Work out the finished part from the listing and answer in its coordinate system (mm). Face numbers are marked on the shaded views. Round coordinates to 2 decimals unless told otherwise and drop trailing zeros. Order: outer loops, then holes, each group sorted by start corner. A loop starts at its lowest first (then second) coordinate and runs counter-clockwise, first axis right, second up. Notation, with made-up numbers: (-30.75, 78.5) - (10.25, 78.5) arc R20 cw to (10.25, 113.5) - close; hole circle Ø4 at (29, 61). An arc over 180 degrees is marked (long way). Use CSV: the item, a comma, the result in double quotes.
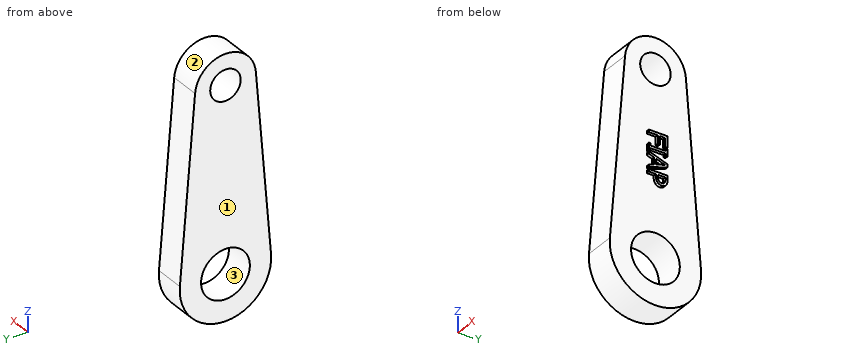
Autodesk Inventor part; units mm, degrees
ref_plane "YZ Plane" through (0, 0, 0) normal (1, 0, 0) x (0, 1, 0)
ref_plane "XZ Plane" through (0, 0, 0) normal (0, 1, 0) x (-1, 0, 0)
ref_plane "XY Plane" through (0, 0, 0) normal (0, 0, 1) x (1, 0, 0)
sketch "Esboço1" plane through (0, 0, 0) normal (1, 0, 0) x (0, 1, 0)
  line L0 (0, 0) -> (0, 30)
  circle A0 centre (0, 0) radius 4
  circle A1 centre (0, 30) radius 2.5
  arc A2 (4.9826, 30.4167) -> (-4.9826, 30.4167) centre (0, 30) ccw
  arc A3 (-7.4739, 0.625) -> (7.4739, 0.625) centre (0, 0) ccw
  line L1 (4.9826, 30.4167) -> (7.4739, 0.625)
  line L2 (-4.9826, 30.4167) -> (-7.4739, 0.625)
extrude "Extrusão1" add sketch "Esboço1" along normal mid plane 5
sketch "Esboço2" plane through (2.5, 0, 0) normal (1, 0, 0) x (0, 0, -1)
  line L0 (-19.9846, 1.6224) -> (-11.4087, 1.6224) construction
  line L1 (-11.4087, 1.6224) -> (-11.4087, -1.4256) construction
  line L2 (-11.4087, -1.4256) -> (-19.9846, -1.4256) construction
  line L3 (-19.9846, -1.4256) -> (-19.9846, 1.6224) construction
  circle A0 centre (-30, 0) radius 2.5
  line L4 (-17.853, 1.2618) -> (-19.2708, 1.2618)
  line L5 (-19.2708, 1.2618) -> (-19.2708, 0.4022)
  line L6 (-19.2708, 0.4022) -> (-17.9122, 0.4022)
  line L7 (-17.9122, 0.4022) -> (-17.9122, 0.0416)
  line L8 (-17.9122, 0.0416) -> (-19.2708, 0.0416)
  line L9 (-19.2708, 0.0416) -> (-19.2708, -1.4256)
  line L10 (-19.2708, -1.4256) -> (-19.6758, -1.4256)
  line L11 (-19.6758, -1.4256) -> (-19.6758, 1.6224)
  line L12 (-19.6758, 1.6224) -> (-17.853, 1.6224)
  line L13 (-17.853, 1.6224) -> (-17.853, 1.2618)
  line L14 (-16.4278, -1.4256) -> (-17.6084, -1.4256)
  line L15 (-17.6084, -1.4256) -> (-17.6084, -1.1144)
  line L16 (-17.6084, -1.1144) -> (-17.2206, -1.1144)
  line L17 (-17.2206, -1.1144) -> (-17.2206, 1.3112)
  line L18 (-17.2206, 1.3112) -> (-17.6084, 1.3112)
  line L19 (-17.6084, 1.3112) -> (-17.6084, 1.6224)
  line L20 (-17.6084, 1.6224) -> (-16.4278, 1.6224)
  line L21 (-16.4278, 1.6224) -> (-16.4278, 1.3112)
  line L22 (-16.4278, 1.3112) -> (-16.8156, 1.3112)
  line L23 (-16.8156, 1.3112) -> (-16.8156, -1.1144)
  line L24 (-16.8156, -1.1144) -> (-16.4278, -1.1144)
  line L25 (-16.4278, -1.1144) -> (-16.4278, -1.4256)
  line L26 (-16.2549, -1.4256) -> (-15.2273, 1.6224)
  line L27 (-15.2273, 1.6224) -> (-14.7284, 1.6224)
  line L28 (-14.7284, 1.6224) -> (-13.7009, -1.4256)
  line L29 (-13.7009, -1.4256) -> (-14.1282, -1.4256)
  line L30 (-14.1282, -1.4256) -> (-14.4048, -0.5735)
  line L31 (-14.4048, -0.5735) -> (-15.5682, -0.5735)
  line L32 (-15.5682, -0.5735) -> (-15.8448, -1.4256)
  line L33 (-15.8448, -1.4256) -> (-16.2549, -1.4256)
  line L34 (-14.516, -0.2276) -> (-14.9877, 1.2074)
  line L35 (-14.9877, 1.2074) -> (-15.457, -0.2276)
  line L36 (-15.457, -0.2276) -> (-14.516, -0.2276)
  spline S0 degree 2 poles (-11.4853, 0.7035) (-11.4853, 0.5059) (-11.6261, 0.1503) (-11.752, 0.0268) knots 0 0 0 1 2 2 2
  spline S1 degree 2 poles (-11.752, 0.0268) (-11.9101, -0.1288) (-12.3374, -0.2894) (-12.6635, -0.2894) knots 0 0 0 1 2 2 2
  line L37 (-12.6635, -0.2894) -> (-13.0068, -0.2894)
  line L38 (-13.0068, -0.2894) -> (-13.0068, -1.4256)
  line L39 (-13.0068, -1.4256) -> (-13.4119, -1.4256)
  line L40 (-13.4119, -1.4256) -> (-13.4119, 1.6224)
  line L41 (-13.4119, 1.6224) -> (-12.6462, 1.6224)
  spline S2 degree 2 poles (-12.6462, 1.6224) (-12.3745, 1.6224) (-11.9941, 1.5335) (-11.8484, 1.4322) knots 0 0 0 1 2 2 2
  spline S3 degree 2 poles (-11.8484, 1.4322) (-11.6779, 1.3161) (-11.4853, 0.958) (-11.4853, 0.7035) knots 0 0 0 1 2 2 2
  spline S4 degree 2 poles (-11.9076, 0.6912) (-11.9076, 0.8493) (-12.0163, 1.0815) (-12.1275, 1.1556) knots 0 0 0 1 2 2 2
  spline S5 degree 2 poles (-12.1275, 1.1556) (-12.2238, 1.2198) (-12.4807, 1.2717) (-12.6709, 1.2717) knots 0 0 0 1 2 2 2
  line L42 (-12.6709, 1.2717) -> (-13.0068, 1.2717)
  line L43 (-13.0068, 1.2717) -> (-13.0068, 0.0564)
  line L44 (-13.0068, 0.0564) -> (-12.7302, 0.0564)
  spline S6 degree 2 poles (-12.7302, 0.0564) (-12.4831, 0.0564) (-12.1793, 0.1354) (-12.0805, 0.2392) knots 0 0 0 1 2 2 2
  spline S7 degree 2 poles (-12.0805, 0.2392) (-11.9891, 0.3306) (-11.9076, 0.5455) (-11.9076, 0.6912) knots 0 0 0 1 2 2 2
  point P0 (0, 0)
extrude "Extrusão2" add sketch "Esboço2" along normal blind 0.5 contours L4 L5 L6 L7 L8 L9 L10 L11 L12 L13 | L14 L15 L16 L17 L18 L19 L20 L21 L22 L23 L24 L25 | L26 L27 L28 L29 L30 L31 L32 L33 | S0 S1 L37 L38 L39 L40 L41 S2 S3
(1) Find the intervals of material crossed by L1, parallel to Y at x = -1.7, z = 0; L2, parallel to Z at x = 0.2, y = 1.5; L3, parallel to X at y = 4.75, z = 6, in increasing order. Write a range as from..to.
Findings below:
L1,"y = -7.5..-4, 4..7.5"
L2,"z = -7.35..-3.71, 3.71..28, 32..34.77"
L3,"x = -2.5..2.5"
(2) Find section D-D (y = -5.5). Determine the outline of the cut face in (x, z), and give its area (3 significant figures).
Findings below:
outline,"(-2.5, -5.1) - (2.5, -5.1) - (2.5, 24.23) - (-2.5, 24.23) - close"
area,"147 mm²"
(3) The mould has two halves that part along Z. Classify the marked faces 1, 2 and 3: released by +Z, released by -Z, zero draft, split by the parting line, or undercut.
Findings below:
face 1,"zero draft"
face 2,"released by +Z"
face 3,"undercut"
(4) Find section A-A (z = 0). Determine the outline of the cut face in (x, y), and give its area (3 significant figures).
Findings below:
outline,"(-2.5, -7.5) - (2.5, -7.5) - (2.5, -4) - (-2.5, -4) - close; (-2.5, 4) - (2.5, 4) - (2.5, 7.5) - (-2.5, 7.5) - close"
area,"35.0 mm²"
(5) Find section C-C (z = 30). Determine the outline of the cut face in (x, y).
Findings below:
outline,"(-2.5, -5.02) - (2.5, -5.02) - (2.5, -2.5) - (-2.5, -2.5) - close; (-2.5, 2.5) - (2.5, 2.5) - (2.5, 5.02) - (-2.5, 5.02) - close"
(6) Each of these flat-tipped pins is pushed along its axis until it touches: pin 1 (1.5 mm diameter, centred on y = 3.5, z = 24.5, fed in from +X); pin 2 (1.5 mm diameter, centred on x = -1.5, y = -5, fed in from +Z); pin 3 (0.5 mm diameter, centred on y = 0.5, z = 15, fed in from +X); pin 4 (0.6 mm diameter, centred on x = 2.5, z = 18.5, fed in from +Y). Where does it stop, or does it pass through?
Findings below:
pin 1,"stops at x = 2.5"
pin 2,"stops at z = 32.63"
pin 3,"stops at x = 3"
pin 4,"stops at y = 6"
(7) Find section B-B (x = 1.15). Determine the outline of the cut face in (y, z) (3 decimals), and give its area (3 significant figures).
Findings below:
outline,"(-7.474, 0.625) arc R7.5 ccw (long way) to (7.474, 0.625) - (4.983, 30.417) arc R5 ccw to (-4.983, 30.417) - close; hole circle Ø8 at (0, 0); hole circle Ø5 at (0, 30)"
area,"434 mm²"
